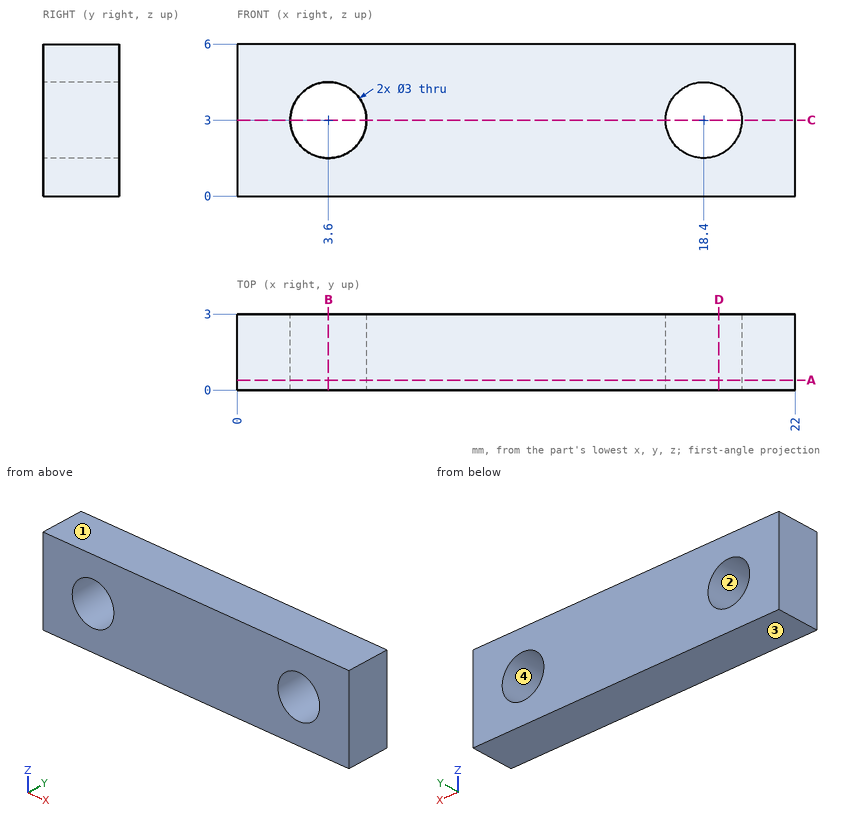
Design review of the part shown in the three views and the two pictorial views. Dimensions are in mm from the part's minimum x, y and z. Coordinates: 2 decimals unless noted, no trailing zeros. Write each loop counter-clockwise with the first axis right and the second up, starting at its lowest first coordinate (ties: lowest second). Pieces come first, ordered by that corner, then holes.
(1) Wall thickness on probe 1 along Z at (x, y) = (18.4, 2.45); probe 2 along X at (y, z) = (1.5, 4.05); probe 3 along X at (y, z) = (1.4, 1.65): over which ranges is each line inside the solid? List them lowest first.
(2) Add section D-D on x = 19. Give the boundary of the cut face in (y, z).
(3) Add section B-B on x = 3.6. Give the boundary of the cut face in (y, z), then the cut area to 3 significant figures.
(4) Add section C-C on z = 3. Give the boundary of the cut face in (x, y), then the cut area to 3 significant figures.
(5) The part is to be moulded in two halves that separate along Z. For the marked faces 1, 2, 3 and 4, say which applies: +Z half, -Z half, draft (parallel to the pull), parting line (faces both ways), or undercut.
(6) Add section A-A on y = 0.4. Give the boundary of the cut face in (x, z), then the cut area to 3 significant figures.
Answer sheet:
1. probe 1: z = 0 to 1.5, 4.5 to 6
1. probe 2: x = 0 to 2.53, 4.67 to 17.33, 19.47 to 22
1. probe 3: x = 0 to 2.95, 4.25 to 17.75, 19.05 to 22
2. outline: (0, 0) - (3, 0) - (3, 1.63) - (0, 1.63) - close; (0, 4.37) - (3, 4.37) - (3, 6) - (0, 6) - close
3. outline: (0, 0) - (3, 0) - (3, 1.5) - (0, 1.5) - close; (0, 4.5) - (3, 4.5) - (3, 6) - (0, 6) - close
3. area: 9.00 mm2
4. outline: (0, 0) - (2.1, 0) - (2.1, 3) - (0, 3) - close; (5.1, 0) - (16.9, 0) - (16.9, 3) - (5.1, 3) - close; (19.9, 0) - (22, 0) - (22, 3) - (19.9, 3) - close
4. area: 48.0 mm2
5. face 1: +Z half
5. face 2: undercut
5. face 3: -Z half
5. face 4: undercut
6. outline: (0, 0) - (22, 0) - (22, 6) - (0, 6) - close; hole circle Ø3 at (3.6, 3); hole circle Ø3 at (18.4, 3)
6. area: 118 mm2
